```python
from build123d import *

# Parameters (mm, degrees)
F0_R     = 5
F1_DEPTH = 30
F3_DEPTH = 8
F4_R     = 1.25
F5_DEPTH = 5
F7_D     = 4
F7_DEPTH = 10
F7_TIP   = 1.2017212381


with BuildPart() as f1:
    # F0 (on Top) → F1 (new body)
    with BuildSketch(Plane.XY):
        Circle(F0_R)
    extrude(amount=F1_DEPTH)

    # F2 (on face) → F3 (cut)
    with BuildSketch(Plane.XY.offset(30)):
        with BuildLine():
            ThreePointArc((1.1, 4.8774993593), (0, 5), (-1.1, 4.8774993593))
            Line((-1.1, 4.8774993593), (-1.1, -4.8774993593))
            ThreePointArc((-1.1, -4.8774993593), (0, -5), (1.1, -4.8774993593))
            Line((1.1, -4.8774993593), (1.1, 4.8774993593))
        make_face()
    extrude(amount=-F3_DEPTH, mode=Mode.SUBTRACT)

    # F4 (on Right) → F5 (cut, symmetric)
    with BuildSketch(Plane.YZ):
        with Locations((0, 27)):
            Circle(F4_R)
    extrude(amount=F5_DEPTH, both=True, mode=Mode.SUBTRACT)

    # F7
    with Locations(Plane(origin=(0, 0, 0), x_dir=(1, 0, 0), z_dir=(0, 0, -1))):
        with Locations((0, 0)):
            Hole(F7_D / 2, depth=F7_DEPTH)
            with Locations((0, 0, -(F7_DEPTH + F7_TIP / 2))):  # 118° drill point
                Cone(0, F7_D / 2, F7_TIP, mode=Mode.SUBTRACT)


solid = f1.part
```
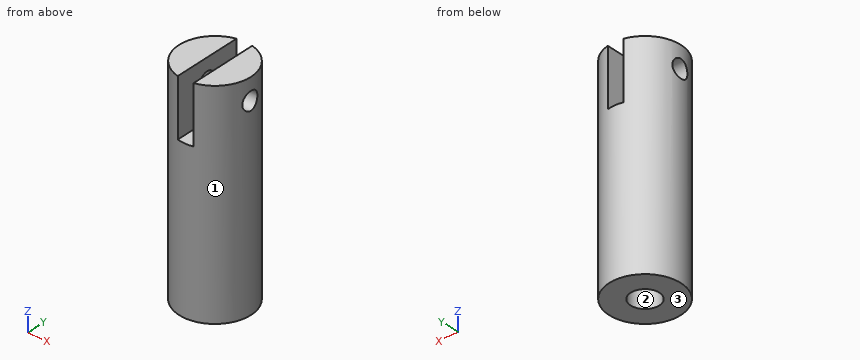
Input: part model. Units: mm. Frame: model coordinates. Face numbers are marked on the shaded views. Round coordinates to 2 decimals unless told otherwise and drop trailing zeros. Order: outer loops, then holes, each group sorted by start corner. A loop starts at its lowest first (then second) coordinate and runs counter-clockwise, first axis right, second up. Notation, with made-up numbers: (77, 48) - (132, 48) arc R15 ccw to (132, 76) - close; hole circle Ø2 at (66, -6). An arc over 180 degrees is marked (long way). Answer in a Markdown table with one row per item.
Item 1: Section query A-A (x = 3). Return the cut outline in (y, z).
Model answer:
| item | result |
|---|---|
| outline | (-4, 0) - (4, 0) - (4, 30) - (-4, 30) - close; hole circle Ø2.5 at (0, 27) |
Item 2: Line query: line 1 (Y direction, x = 0, z = 6.25); line 2 (Z direction, x = 2.25, y = 0); line 3 (Y direction, x = -1.95, z = 27). Output: solid intervals per line, ascending.
Model answer:
| item | result |
|---|---|
| line 1 | y = -5 to -2, 2 to 5 |
| line 2 | z = 0 to 25.75, 28.25 to 30 |
| line 3 | y = -4.6 to -1.25, 1.25 to 4.6 |
Item 3: Pin query (flat end, axial travel): pin 1 (2 mm diameter, centred on y = -2, z = 22, fed in from +X); pin 2 (1 mm diameter, centred on x = -1.5, z = 4.5, fed in from +Y). Return the tip coordinate at first contact, or that it passes through.
Model answer:
| item | result |
|---|---|
| pin 1 | stops at x = 4.9 |
| pin 2 | stops at y = 4.9 |
Item 4: Section query C-C (y = 3). Return the cut outline in (x, z).
Model answer:
| item | result |
|---|---|
| outline | (-4, 0) - (4, 0) - (4, 30) - (1.1, 30) - (1.1, 22) - (-1.1, 22) - (-1.1, 30) - (-4, 30) - close |
Item 5: Section query B-B (z = 27). Return the cut outline in (x, y), then the cut area to 3 significant figures.
Model answer:
| item | result |
|---|---|
| outline | (-4.84, -1.25) arc R5 ccw to (-1.1, -4.88) - (-1.1, -1.25) - close; (-4.84, 1.25) - (-1.1, 1.25) - (-1.1, 4.88) arc R5 ccw to start; (1.1, -4.88) arc R5 ccw to (4.84, -1.25) - (1.1, -1.25) - close; (1.1, 1.25) - (4.84, 1.25) arc R5 ccw to (1.1, 4.88) - close |
| area | 37.5 mm² |
Item 6: Section query D-D (z = 8.5). Return the cut outline in (x, y), then the cut area to 3 significant figures.
Model answer:
| item | result |
|---|---|
| outline | circle Ø10 at (0, 0); hole circle Ø4 at (0, 0) |
| area | 66.0 mm² |
Item 7: Mould query, pull axis Y, two halves, no side actions, for the marked faces 1, 2 and 3. Classes: released by +Y, released by -Y, zero draft, split by the parting line, or undercut.
Model answer:
| item | result |
|---|---|
| face 1 | split by the parting line |
| face 2 | undercut |
| face 3 | zero draft |
